Can you work these out from the model? Positions are in its coordinate system, mm. Face numbers are marked on the shaded views. Round coordinates to 2 decimals unless told otherwise and drop trailing zeros. Write each loop counter-clockwise with the first axis right and the second up, starting at its lowest first coordinate (ties: lowest second). Pieces come first, ordered by that corner, then holes.
Q1. Please list where these lines run through material, in increasing order: line 1 along Z through (x, y) = (57.3, 3.95); line 2 along X through (y, z) = (2.8, -12.5); line 3 along Z through (x, y) = (68.75, 2.5).
Q2. We'd pull the mould along Z, two halves only. Please class the marked faces 1 and 2: +Z half, -Z half, draft (parallel to the pull), parting line (faces both ways), or undercut.
Q3. If we section it at A-A (z = -12.5): Please give me the cut outline in (x, y), plus the area to 3 significant figures.
Q4. I'm going to push flat-ended pins straight in: pin 1 Ø2 at (x, z) = (64.3, -12.5) entering from +Y; pin 2 Ø1.5 at (y, z) = (2.5, -4) entering from +X. Where does each tip first touch, or does it pass through?
Q5. If we section it at C-C (z = -36): Please give me the cut outline in (x, y), plus the area to 3 significant figures.
Q6. If we section it at B-B (x = 11): Please give me the cut outline in (y, z), plus the area to 3 significant figures.
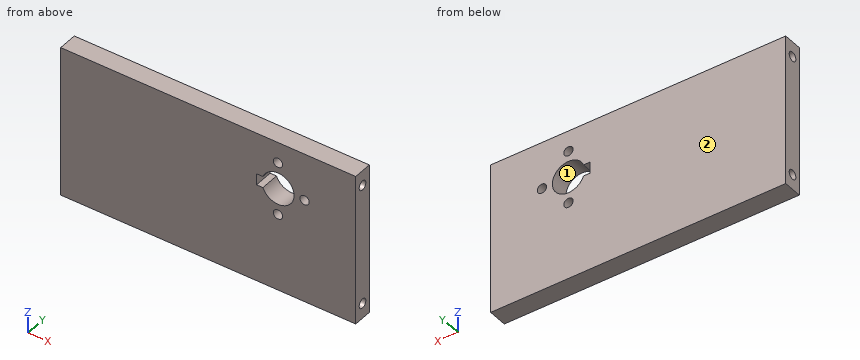
Autodesk Inventor part; units mm, degrees
ref_plane "YZ Plane" through (0, 0, 0) normal (1, 0, 0) x (0, 1, 0)
ref_plane "XZ Plane" through (0, 0, 0) normal (0, 1, 0) x (-1, 0, 0)
ref_plane "XY Plane" through (0, 0, 0) normal (0, 0, 1) x (1, 0, 0)
sketch "スケッチ2" plane through (0, 0, 0) normal (0, 1, 0) x (-1, 0, 0)
  line L0 (0, 0) -> (-77.8, 0)
  line L1 (-77.8, 0) -> (-77.8, -40)
  line L2 (-77.8, -40) -> (0, -40)
  line L3 (0, -40) -> (0, 0)
  dimension "d0" = 77.8
  dimension "d1" = 40
extrude "押し出し1" add sketch "スケッチ2" along normal blind 5
sketch "スケッチ4" plane through (0, 0, -40) normal (-1, 0, 0) x (0, 0, 1)
  line L0 (0, 0) -> (0, 5) construction
  line L1 (0, 2.5) -> (40, 2.5) construction
  line L2 (40, 0) -> (40, 5) construction
  point P0 (4, 2.5)
  point P1 (36, 2.5)
  dimension "d4" = 4
  dimension "d5" = 4
hole "穴1" at (0, 2.5, -36) at (0, 2.5, -4) direction (1, 0, 0) diameter 2.459 depth 12
sketch "スケッチ5" plane through (77.8, 0, 0) normal (1, 0, 0) x (0, 0, -1)
  line L0 (0, 0) -> (0, 5) construction
  line L1 (0, 2.5) -> (39.9198, 2.5) construction
  circle A0 centre (4, 2.5) radius 1.2295 construction
  circle A1 centre (36, 2.5) radius 1.2295
  point P0 (4, 2.5)
  point P1 (36, 2.5)
hole "穴2" at (77.8, 2.5, -4) at (77.8, 2.5, -36) direction (-1, 0, 0) diameter 2.459 depth 13
sketch "スケッチ6" plane through (0, 5, 0) normal (0, 1, 0) x (1, 0, 0)
  line L0 (77.8, 0) -> (77.8, 40) construction
  line L1 (0, 40) -> (0, 0) construction
  line L2 (0, 0) -> (77.8, 0) construction
  point P0 (57.3, 12.5)
  dimension "d20" = 20.5
  dimension "d21" = 12.5
hole "穴3" at (57.3, 5, -12.5) direction (0, -1, 0) diameter 8.5 end through all
sketch "スケッチ7" plane through (0, 5, 0) normal (0, 1, 0) x (1, 0, 0)
  line L0 (77.8, 0) -> (77.8, 40) construction
  line L1 (77.8, 28.3) -> (0, 28.3) construction
  line L2 (0, 40) -> (0, 0) construction
  circle A0 centre (57.3, 12.5) radius 4.25 construction
  point P0 (67.8, 28.3)
  point P1 (46.8, 28.3)
  dimension "d29" = 15.8
  dimension "d30" = 10.5
  dimension "d31" = 10.5
hole "穴4" [suppressed]
sketch "スケッチ8" plane through (0, 5, 0) normal (0, 1, 0) x (1, 0, 0)
  circle A0 centre (57.3, 12.5) radius 4.25 construction
  circle A1 centre (57.3, 12.5) radius 7 construction
  point P0 (0, 0)
  point P1 (64.3, 12.5)
  point P2 (57.3, 19.5)
  point P3 (57.3, 5.5)
  dimension "d39" = 14
hole "穴5" at (64.3, 5, -12.5) at (57.3, 5, -19.5) at (57.3, 5, -5.5) direction (0, -1, 0) diameter 2.459 end through all
sketch "スケッチ9" plane through (0, 5, 0) normal (0, 1, 0) x (1, 0, 0)
  circle A0 centre (57.3, 12.5) radius 4.25
  line L0 (57.3, 12.5) -> (45.9478, 12.5) construction
  line L1 (51.65, 14) -> (53.05, 14)
  line L2 (53.05, 14) -> (53.05, 11)
  line L3 (53.05, 11) -> (51.65, 11)
  line L4 (51.65, 11) -> (51.65, 14)
  line L5 (51.65, 14) -> (53.05, 11) construction
  line L6 (53.05, 14) -> (51.65, 11) construction
  line L7 (53.05, 11) -> (53.3235, 11)
  line L8 (53.05, 14) -> (53.3235, 14)
  point P0 (0, 0)
  point P1 (52.35, 12.5)
  dimension "d56" = 1.4
  dimension "d57" = 0
  dimension "d58" = 3
extrude "押し出し2" cut sketch "スケッチ9" against normal blind 10 contours A0 L2 L8 | L7 L2 A0 | L2 L3 L4 L1
properties part number "shoulder1_verticval_right_cover" material "アルミニウム 5052"
A:
1. line 1: z = -40 to -20.73, -18.27 to -16.75, -8.25 to -6.73, -4.27 to 0
1. line 2: x = 0 to 51.65, 61.55 to 63.07, 65.53 to 77.8
1. line 3: z = -40 to -37.23, -34.77 to -5.23, -2.77 to 0
2. face 1: undercut
2. face 2: draft
3. outline: (0, 0) - (51.65, 0) - (51.65, 5) - (0, 5) - close; (61.55, 0) - (63.07, 0) - (63.07, 5) - (61.55, 5) - close; (65.53, 0) - (77.8, 0) - (77.8, 5) - (65.53, 5) - close
3. area: 327 mm2
4. pin 1: passes through
4. pin 2: stops at x = 64.8
5. outline: (0, 0) - (77.8, 0) - (77.8, 1.27) - (64.8, 1.27) - (64.8, 3.73) - (77.8, 3.73) - (77.8, 5) - (0, 5) - (0, 3.73) - (12, 3.73) - (12, 1.27) - (0, 1.27) - close
5. area: 328 mm2
6. outline: (0, -40) - (5, -40) - (5, 0) - (0, 0) - close; hole circle Ø2.46 at (2.5, -36); hole circle Ø2.46 at (2.5, -4)
6. area: 191 mm2
